Model file for the job. Use its own axes, mm. Give positions to 0.01 mm unless a question says otherwise; leave off trailing zeros. Order: outer loops, then holes, each group sorted by start corner. A loop starts at its lowest first (then second) coordinate and runs counter-clockwise, first axis right, second up. Notation, with made-up numbers: (-18, 5) -> (-1, 5) arc R19 cw to (-1, 26) -> close; hole circle Ø8 at (-5.5, 17). An arc over 180 degrees is marked (long way). Use CSV: the item, a comma, the result in double quotes. Start each with the question number.
1. Cut at C-C on y = -30.5. List the corners of the cut face in (x, z), then the cut area to 3 significant figures.
2. Cut at A-A on x = 140.5. List the corners of the cut face in (y, z).
3. Cut at B-B on z = 1.65. List the corners of the cut face in (x, y), then the cut area to 3 significant figures.
4. Wall check: line 1 (Y direction, x = 124.5, z = 0.2); line 2 (X direction, y = -14, z = 1.3). Give the ranges that are in metal, low to high. Write a range as from..to.
Autodesk Inventor part; units mm, degrees
ref_plane "YZ Plane" through (0, 0, 0) normal (1, 0, 0) x (0, 1, 0)
ref_plane "XZ Plane" through (0, 0, 0) normal (0, 1, 0) x (-1, 0, 0)
ref_plane "XY Plane" through (0, 0, 0) normal (0, 0, 1) x (1, 0, 0)
sketch "Sketch1" plane through (0, 0, 0) normal (0, 0, 1) x (1, 0, 0)
  line L0 (0, -255.5) -> (700, -255.5)
  line L1 (700, -255.5) -> (700, 255.5)
  line L2 (700, 255.5) -> (0, 255.5)
  line L3 (0, 255.5) -> (0, -255.5)
  point P0 (0, 0)
  point P1 (0, 0)
  dimension "d0" = 700
  dimension "d1" = 511
extrude "Plate1" add sketch "Sketch1" along normal blind 3
sketch "Sketch6" plane through (0, 0, 3) normal (0, 0, 1) x (1, 0, 0)
  line L0 (0, -255.5) -> (700, -255.5)
  line L1 (0, -255.5) -> (300, -255.5)
  line L2 (300, -255.5) -> (300, 44.5)
  line L3 (300, 44.5) -> (0, 44.5)
  line L4 (0, 44.5) -> (0, -255.5)
  point P0 (0, 0)
  dimension "d36" = 300
  dimension "d37" = 300
extrude "Extrusion2" cut sketch "Sketch6" against normal up to surface (3 mm away)
equation "\"d2\" = Thickness"
equation "\"BendReliefWidth\" = Thickness"
equation "\"BendReliefDepth\" = 0.5 * Thickness"
equation "\"CornerReliefSize\" = 4 * Thickness"
equation "\"MinimumRemnant\" = 2 * Thickness"
equation "\"TransitionRadius\" = BendRadius"
equation "\"JacobiRadiusSize\" = BendRadius"
equation "\"GapSize\" = Thickness"
properties part number "BSH 053 sheet in" material "09g2s"
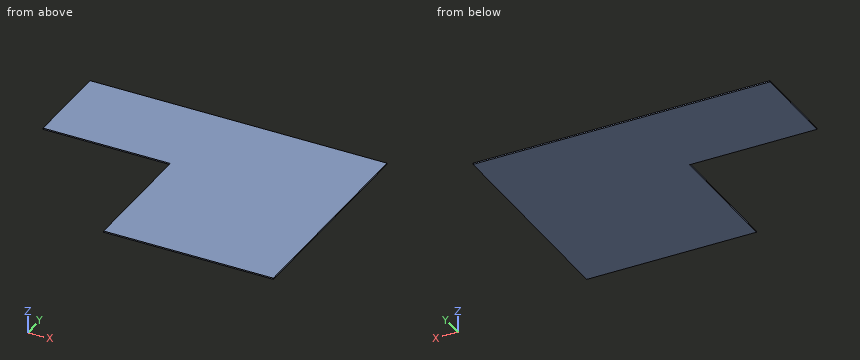
Verdict:
1,outline,"(300, 0) -> (700, 0) -> (700, 3) -> (300, 3) -> close"
1,area,"1,200 mm^2"
2,outline,"(44.5, 0) -> (255.5, 0) -> (255.5, 3) -> (44.5, 3) -> close"
3,outline,"(0, 44.5) -> (300, 44.5) -> (300, -255.5) -> (700, -255.5) -> (700, 255.5) -> (0, 255.5) -> close"
3,area,"268,000 mm^2"
4,line 1,"44.5..255.5"
4,line 2,"300..700"
